from build123d import *

# Parameters (mm, degrees)
BOSS_EXTRUDE1_DEPTH = 95.25
SKETCH2_R           = 3.175
CUT_EXTRUDE1_DEPTH  = 152.4
SKETCH4_R           = 34.925
SKETCH4_R_2         = 3.81
CUT_EXTRUDE2_DEPTH  = 381
SKETCH5_R           = 3.81
CUT_EXTRUDE3_DEPTH  = 12.7
SKETCH6_W           = 473.075
SKETCH6_H           = 95.25
CUT_EXTRUDE4_DEPTH  = 3.175


with BuildPart() as part:
    # Sketch1 → Boss-Extrude1 (new body)
    with BuildSketch(Plane.XY):
        Polygon((0, 0), (0, 381), (3.175, 381), (3.175, 3.175), (473.075, 3.175), (473.075, 0), align=None)
    extrude(amount=BOSS_EXTRUDE1_DEPTH)

    # Sketch2 → Cut-Extrude1 (cut)
    with BuildSketch(Plane(origin=(0, 3.175, 0), x_dir=(1, 0, 0), z_dir=(0, 1, 0))):
        with Locations(Location((190.119, -4.572, 0), (0, 0, 180))):
            Circle(SKETCH2_R)
        with Locations(Location((190.119, -76.2, 0), (0, 0, 180))):
            Circle(SKETCH2_R)
        with Locations(Location((261.747, -4.572, 0), (0, 0, 180))):
            Circle(SKETCH2_R)
        with Locations(Location((261.747, -76.2, 0), (0, 0, 180))):
            Circle(SKETCH2_R)
        with Locations(Location((295.783, -76.2, 0), (0, 0, 180))):
            Circle(SKETCH2_R)
        with Locations(Location((295.783, -4.572, 0), (0, 0, 180))):
            Circle(SKETCH2_R)
        with Locations(Location((367.411, -76.2, 0), (0, 0, 180))):
            Circle(SKETCH2_R)
        with Locations(Location((367.411, -4.572, 0), (0, 0, 180))):
            Circle(SKETCH2_R)
    extrude(amount=-CUT_EXTRUDE1_DEPTH, mode=Mode.SUBTRACT)

    # Sketch4 → Cut-Extrude2 (cut)
    with BuildSketch(Plane.XZ):
        with Locations((225.933, 40.386)):
            Circle(SKETCH4_R)
        with Locations((331.597, 40.386)):
            Circle(SKETCH4_R)
        with Locations((390.525, 19.05)):
            Circle(SKETCH4_R_2)
    extrude(amount=-CUT_EXTRUDE2_DEPTH, mode=Mode.SUBTRACT)

    # Sketch5 → Cut-Extrude3 (cut)
    with BuildSketch(Plane.ZY):
        with Locations((19.05, 349.25)):
            Circle(SKETCH5_R)
    extrude(amount=-CUT_EXTRUDE3_DEPTH, mode=Mode.SUBTRACT)

    # Sketch6 → Cut-Extrude4 (cut)
    with BuildSketch(Plane.XZ):
        with Locations((236.5375, 47.625)):
            Rectangle(SKETCH6_W, SKETCH6_H)
    extrude(amount=-CUT_EXTRUDE4_DEPTH, mode=Mode.SUBTRACT)


solid = part.part
Here's how the part is built. I have some questions about the finished solid (model axes, mm). Give positions to 0.01 mm unless a question says otherwise; leave off trailing zeros. Loops run counter-clockwise (first coordinate to the right, second up) from the corner with the lowest first, then second, coordinate; pieces in that order, holes last. Notation, with made-up numbers: (-30.5, 1) -> (-18.5, 1) arc R20 cw to (-18.5, 7) -> close; hole circle Ø8 at (76.25, 30). An arc over 180 degrees is marked (long way). Answer as a JSON object with one key per item and string values. Group by question number.
Item 1: Thinking about a two-plate mould opening in Z: for faces 1 (the flat face through (3.175, 195, 47)), 2 (the cylindrical face through (1.57, 345.53, 18.22)), which applies, pulls with the +Z half, pulls with the -Z half, needs draft (parallel to the pull), parting line crosses it, or undercut?
Item 2: I need wall thicknesses on L1, parallel to Z at x = 1.3, y = 349.25; L2, parallel to Y at x = 2.45, z = 19.05 (3 decimals). Which ranges of each line are inside material? Lowest first, please.
Item 3: Imagine slicing it at B-B on z = 19.05. Write out the boundary of the cut face in (x, y) (3 decimals).
Item 4: Imagine slicing it at A-A on y = 349.25. Write out the boundary of the cut face in (x, z) (3 decimals).
Answer list:
{
 "1": {"face 1": "needs draft", "face 2": "undercut"},
 "2": {"L1": "z = 0 to 15.24, 22.86 to 95.25", "L2": "y = 3.175 to 345.44, 353.06 to 381"},
 "3": {"outline": "(0, 3.175) -> (3.175, 3.175) -> (3.175, 345.44) -> (0, 345.44) -> close; (0, 353.06) -> (3.175, 353.06) -> (3.175, 381) -> (0, 381) -> close"},
 "4": {"outline": "(0, 0) -> (3.175, 0) -> (3.175, 15.24) -> (0, 15.24) -> close; (0, 22.86) -> (3.175, 22.86) -> (3.175, 95.25) -> (0, 95.25) -> close"}
}
